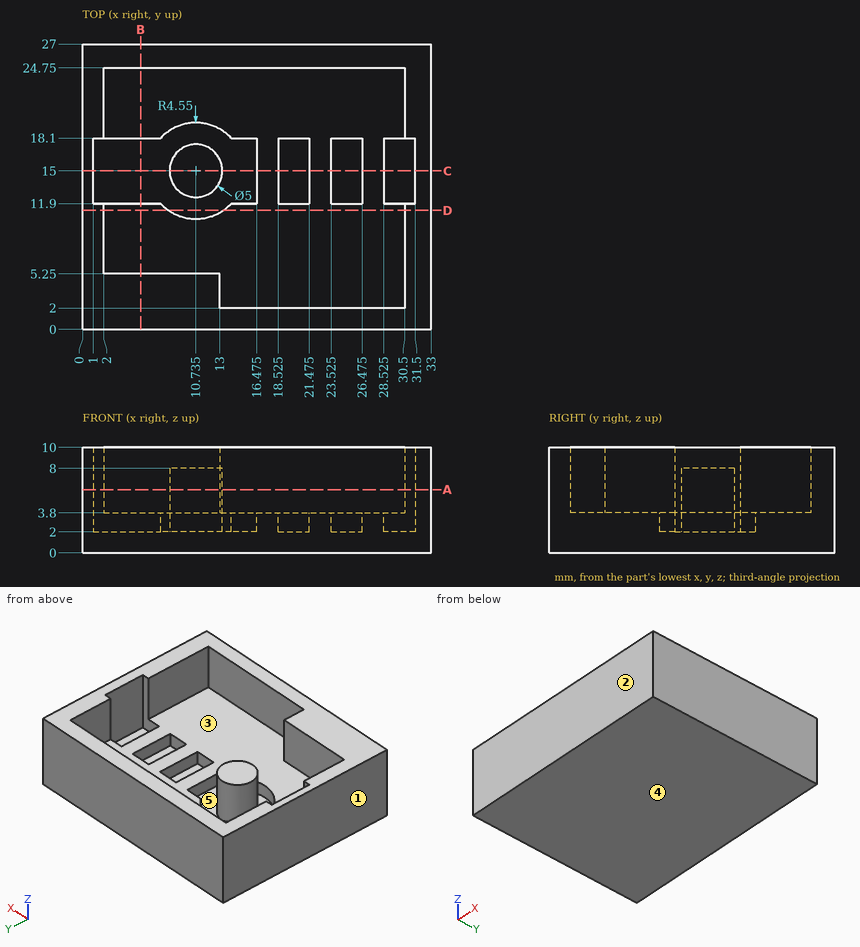
Drawing for the job (mm, zero at the part's lowest x, y, z). A direction names the side the tool comes from. Give positions to 0.01 mm unless a question says otherwise; leave off trailing zeros. Order: outer loops, then holes, each group sorted by start corner. A loop starts at its lowest first (then second) coordinate and runs counter-clockwise, first axis right, second up. Notation, with made-up numbers: M 51,-34 L 101,-34 A27 ccw 101,-16 Z; hole C 31,84.25 d6. An arc over 180 degrees is marked long. Put each result on its own line as item: value.
Item 1: Two-plate mould, pull along X, no slides. Class the marked faces 1, 2 and 3: +X half, -X half, draft (parallel to the pull), parting line (faces both ways), or undercut.
From the geometry:
face 1: -X half
face 2: draft
face 3: undercut
Item 2: Slice it at C-C, the plane y = 15. Write the cut outline in (x, z) (3 decimals).
From the geometry:
outline: M 0,0 L 33,0 L 33,10 L 31.5,10 L 31.5,2 L 28.525,2 L 28.525,3.8 L 26.475,3.8 L 26.475,2 L 23.525,2 L 23.525,3.8 L 21.475,3.8 L 21.475,2 L 18.525,2 L 18.525,3.8 L 16.475,3.8 L 16.475,2 L 13.235,2 L 13.235,8 L 8.235,8 L 8.235,2 L 1,2 L 1,10 L 0,10 Z
Item 3: Probe line 1 (X direction, y = 2.5, z = 8.25); line 2 (Y direction, x = 16.5, z = 8.5); line 3 (X direction, y = 12.25, z = 8.25). List the from-to ranges inside material, lowest first. Write a range as [from, to].
From the geometry:
line 1: x = [0, 13], [30.5, 33]
line 2: y = [0, 2], [24.75, 27]
line 3: x = [0, 1], [31.5, 33]
Item 4: Slice it at A-A, the plane z = 6. Write the cut outline in (x, y) (3 decimals).
From the geometry:
outline: M 0,0 L 33,0 L 33,27 L 0,27 Z; C 10.735,15 d5; hole M 1,11.9 L 2,11.9 L 2,5.25 L 13,5.25 L 13,2 L 30.5,2 L 30.5,11.9 L 31.5,11.9 L 31.5,18.1 L 30.5,18.1 L 30.5,24.75 L 2,24.75 L 2,18.1 L 1,18.1 Z
Item 5: Slice it at B-B, the plane x = 5.5. Write the cut outline in (y, z).
From the geometry:
outline: M 0,0 L 27,0 L 27,10 L 24.75,10 L 24.75,3.8 L 18.1,3.8 L 18.1,2 L 11.9,2 L 11.9,3.8 L 5.25,3.8 L 5.25,10 L 0,10 Z
Item 6: Flat gauge pins, fed straight in: pin 1 Ø2.5 at (x, y) = (19.5, 14) entering from +Z; pin 2 Ø1.5 at (x, y) = (30.5, 16.5) entering from +Z. Where does each tip first touch, or does it go through?
From the geometry:
pin 1: stops at z = 3.8
pin 2: stops at z = 2
Item 7: Slice it at D-D, the plane y = 11.25. Write the cut outline in (x, z), plus the area to 3 significant figures.
From the geometry:
outline: M 0,0 L 33,0 L 33,10 L 30.5,10 L 30.5,3.8 L 13.31,3.8 L 13.31,2 L 8.16,2 L 8.16,3.8 L 2,3.8 L 2,10 L 0,10 Z
area: 144 mm2
Item 8: 3-axis set-ups, long thin cutter, end or side, ignore diameter. For the marked faces 4 and 5: which of +Z, -Z, +X, -X, +Y, -Y reach the whole face in a straight line?
From the geometry:
face 4: -Z, +X, -X, +Y, -Y
face 5: +Z
